The model under review builds one solid part; all positions refer to its coordinate system, in mm. A direction names the side the tool comes from. Coordinates: 2 decimals unless noted, no trailing zeros. Loops run counter-clockwise (first coordinate to the right, second up) from the corner with the lowest first, then second, coordinate; pieces in that order, holes last. Notation, with made-up numbers: (84.25, 85) - (95.25, 85) arc R18 cw to (95.25, 102) - close; hole circle Ø6 at (17, 55.5). An arc over 180 degrees is marked (long way). One line per item, written item: value. Start each with the question number.
1. We need section D-D, the plane z = -19. Give the boundary of the cut face in (x, y).
2. We need section A-A, the plane y = 3.75. Give the boundary of the cut face in (x, z).
3. To check wall thickness, follow line 1 (Y direction, x = -13, z = 0.5); line 2 (Z direction, x = -8, y = 3.75); line 3 (X direction, y = 3.5, z = 7). State the ranges of each line that lie inside material, in increasing order.
4. Mouldability with a two-part tool opening along X and no side actions: class faces 1 (the face through (0, 5.08, 3)), 2 (the face through (1.27, 11, 18)), 3 (the face through (-20.3, 5.52, -12.37)) as +X half, -X half, draft (parallel to the pull), parting line (faces both ways), or undercut.
5. We need section C-C, the plane x = 3. Give the boundary of the cut face in (y, z).
6. For faces 4 (the face through (0, 10, 21.59)), 5 (the face through (-13.823, 10.124, -8.671)), 6 (the face through (-17.24, 10.89, -9.2)), 7 (the face through (15.306, 5.523, -12.291)), list the 3-axis set-ups (+Z, -Z, +X, -X, +Y, -Y) from which the entire face can be reached by the end or side of a thin tool; tool diameter is ignored.
7. Insertion check: P1, Ø3, axis at y = 12, z = 19, coming from the +X side; P2, Ø10, axis at x = -11, z = 17, coming from the +Y side; P3, Ø0.8, axis at x = 0, y = 10.5, coming from the +Z side; P4, Ø2.5, axis at y = 12.7, z = 18.415, coming from the -X side. Each pin has a flat end and moves straight along its axis. Give the tip position at first contact, or say it passes through.
8. We need section B-B, the plane z = 19. Give the boundary of the cut face in (x, y).
from build123d import *

# Parameters (mm, degrees)
SKETCH2_R                = 25.4
BOSS_EXTRUDE1_DEPTH      = 5.08
SKETCH3_R                = 1.5
BOSS_EXTRUDE2_DEPTH      = 1.27
FILLET1_R                = 2.54
CIRPATTERN1_COUNT        = 3
FILLET1_OF_CIRPATTERN1_R = 2.54


with BuildPart() as part:
    # Sketch2 → Boss-Extrude1 (new body)
    with BuildSketch(Plane(origin=(0, 0, 0), x_dir=(1, 0, 0), z_dir=(0, 1, 0))):
        Circle(SKETCH2_R)
        with BuildLine():
            ThreePointArc((-14.929745343, 20.549031704), (-2.12e-07, 25.4), (14.929745, 20.549031953))
            Line((14.929745, 20.549031953), (0, 31.396126628))
            Line((0, 31.396126628), (-14.929745343, 20.549031704))
        make_face()
        with BuildLine():
            ThreePointArc((-24.156835493, -7.84903172), (-24.156835512, 7.849031664), (-14.929745343, 20.549031704))
            Line((-14.929745343, 20.549031704), (-29.859490816, 9.701936686))
            Line((-29.859490816, 9.701936686), (-24.156835493, -7.84903172))
        make_face()
        with BuildLine():
            Line((-18.454180211, -25.4), (-1.11e-07, -25.4))
            ThreePointArc((-1.11e-07, -25.4), (-14.929745427, -20.549031644), (-24.156835493, -7.84903172))
            Line((-24.156835493, -7.84903172), (-18.454180211, -25.4))
        make_face()
        with BuildLine():
            Line((18.454180211, -25.4), (24.156835424, -7.849031932))
            ThreePointArc((24.156835424, -7.849031932), (14.929745246, -20.549031775), (-1.11e-07, -25.4))
            Line((-1.11e-07, -25.4), (18.454180211, -25.4))
        make_face()
        with BuildLine():
            Line((24.156835424, -7.849031932), (29.859490816, 9.701936686))
            Line((29.859490816, 9.701936686), (14.929745, 20.549031953))
            ThreePointArc((14.929745, 20.549031953), (22.6315656, 11.531358918), (25.4, 0))
            ThreePointArc((25.4, 0), (25.087283828, -3.973435555), (24.156835424, -7.849031932))
        make_face()
    extrude(amount=BOSS_EXTRUDE1_DEPTH)

    # Sketch3 → Boss-Extrude2 (add, symmetric)
    with BuildSketch(Plane(origin=(0, 0, 0), x_dir=(0, 0, -1), z_dir=(1, 0, 0))):
        with BuildLine():
            Line((-21.59, 12.7), (-21.59, 5.08))
            Line((-21.59, 5.08), (-15.24, 5.08))
            Line((-15.24, 5.08), (-15.24, 12.7))
            ThreePointArc((-15.24, 12.7), (-18.415, 15.875), (-21.59, 12.7))
        make_face()
        with Locations((-18.415, 12.7)):
            Circle(SKETCH3_R, mode=Mode.SUBTRACT)
    boss_extrude2 = extrude(amount=BOSS_EXTRUDE2_DEPTH, both=True)

    # Fillet1
    fillet1_edges = [part.edges().sort_by_distance(p)[0] for p in [
        (0, 5.08, 15.24),
        (-1.27, 5.08, 18.415),
        (0, 5.08, 21.59),
        (1.27, 5.08, 18.415),
    ]]
    fillet(fillet1_edges, radius=FILLET1_R)

    # CirPattern1: Boss-Extrude2 ×3 about axis
    cirpattern1_axis = Axis((0, 0, -0.710757359), (0, 1, 0))
    for i in range(1, CIRPATTERN1_COUNT):
        add(boss_extrude2.rotate(cirpattern1_axis, i * 360 / CIRPATTERN1_COUNT))

    # Fillet1 of CirPattern1
    fillet1_of_cirpattern1_edges = [part.edges().sort_by_distance(p)[0] for p in [
        (13.813761083, 5.08, -8.686136039),
        (17.19839174, 5.08, -9.173783776),
        (19.313022397, 5.08, -11.861136039),
        (15.92839174, 5.08, -11.373488302),
        (-13.813761083, 5.08, -8.686136039),
        (-15.92839174, 5.08, -11.373488302),
        (-19.313022397, 5.08, -11.861136039),
        (-17.19839174, 5.08, -9.173783776),
    ]]
    fillet(fillet1_of_cirpattern1_edges, radius=FILLET1_OF_CIRPATTERN1_R)


solid = part.part
Findings below:
1. outline: (-17.06, 0) - (17.06, 0) - (17.06, 5.08) - (-17.06, 5.08) - close
2. outline: (-29.86, -9.7) - (0, -31.4) - (29.86, -9.7) - (18.45, 25.4) - (-18.45, 25.4) - close
3. line 1: 0 to 5.08
3. line 2: -25.58 to 25.4
3. line 3: -24.43 to 24.43
4. face 1: undercut
4. face 2: +X half
4. face 3: -X half
5. outline: (0, -29.22) - (5.08, -29.22) - (5.08, 12.7) arc R2.54 cw to (5.21, 13.51) - (5.21, 23.32) arc R2.54 cw to (5.08, 24.13) - (5.08, 25.4) - (0, 25.4) - close
6. face 4: +Z, +X, -X, +Y
6. face 5: +Z, +Y
6. face 6: +Z, -X, +Y
6. face 7: -Z, +Y
7. P1: x = 1.27
7. P2: y = 5.08
7. P3: z = 21.59
7. P4: through
8. outline: (-20.53, 0) - (20.53, 0) - (20.53, 5.08) - (3.81, 5.08) arc R2.54 cw to (1.27, 7.62) - (1.27, 11.32) - (-1.27, 11.32) - (-1.27, 7.62) arc R2.54 cw to (-3.81, 5.08) - (-20.53, 5.08) - close; (-1.27, 14.08) - (1.27, 14.08) - (1.27, 15.82) - (-1.27, 15.82) - close
